```python
from build123d import *


with BuildPart() as part:
    # Sketch1 → Revolve1 (revolve)
    with BuildSketch(Plane.XY):
        with BuildLine():
            Line((-26.9875, 9.525), (26.9875, 9.525))
            Line((26.9875, 9.525), (26.9875, 19.05))
            Line((26.9875, 19.05), (6.112639692, 19.05))
            Line((6.112639692, 19.05), (6.112639692, 56.974587415))
            Line((6.112639692, 56.974587415), (76.2, 88.9))
            Line((76.2, 88.9), (76.2, 139.7))
            ThreePointArc((76.2, 139.7), (61.321024484, 175.621024484), (25.4, 190.5))
            Line((25.4, 190.5), (-25.4, 190.5))
            ThreePointArc((-25.4, 190.5), (-61.321024484, 175.621024484), (-76.2, 139.7))
            Line((-76.2, 139.7), (-76.2, 88.9))
            Line((-76.2, 88.9), (-6.112639692, 56.974587415))
            Line((-6.112639692, 56.974587415), (-6.112639692, 19.05))
            Line((-6.112639692, 19.05), (-26.9875, 19.05))
            Line((-26.9875, 19.05), (-26.9875, 9.525))
        make_face()
    revolve(axis=Axis((-76.2, 0, 0), (1, 0, 0)))


solid = part.part
```
Could you check a few things on this model? Use its own coordinates, in mm. A direction names the side the tool comes from. Coordinates: 2 decimals unless noted, no trailing zeros. Write each loop counter-clockwise with the first axis right and the second up, starting at its lowest first coordinate (ties: lowest second). Pieces come first, ordered by that corner, then holes. Notation, with made-up numbers: (-21, 79) - (-1, 79) arc R20 ccw to (-1, 114) - close; hole circle Ø8 at (64.5, -21). An arc over 180 degrees is marked (long way). Use a Markdown table: item, result.
Q1. Imagine slicing it at D-D (x = 51). List the corners of the cut face in (y, z) for me, and give its area (3 significant figures).
Geometry check:
| item | result |
|---|---|
| outline | circle Ø367.16 at (0, 0); hole circle Ø154.84 at (0, 0) |
| area | 87,000 mm2 |
Q2. Thinking about a two-plate mould opening in Y: for faces 1 (the conical face through (10.5, -12.78, -57.57)), 2 (the flat face through (76.2, 2, -91)), 3 (the conical face through (-9.516, -46.443, -35.611)), 4 (the cylindrical face through (-0.36, -151.17, -115.92)), which applies, +Y half, -Y half, draft (parallel to the pull), parting line (faces both ways), or undercut?
Geometry check:
| item | result |
|---|---|
| face 1 | undercut |
| face 2 | draft |
| face 3 | undercut |
| face 4 | parting line |
Q3. Imagine slicing it at C-C (x = 0.5). List the corners of the cut face in (y, z) for me (3 decimals).
Geometry check:
| item | result |
|---|---|
| outline | circle Ø381 at (0, 0); hole circle Ø19.05 at (0, 0) |
Q4. I'm going to push flat-ended pins straight in: pin 1 Ø19 at (y, z) = (2, 1) entering from -X; pin 2 Ø3 at (x, z) = (29, 138.5) entering from -Y; pin 3 Ø12 at (x, y) = (49.5, 69) entering from +Z. Where does each tip first touch, or does it pass through?
Geometry check:
| item | result |
|---|---|
| pin 1 | stops at x = -26.99 |
| pin 2 | stops at y = -132.19 |
| pin 3 | stops at z = 174.87 |
Q5. Which directions (+Z, -Z, +X, -X, +Y, -Y) give clear straight access to the entire face, cutting with the end or side of a thin tool? Please do faces 5 (the flat face through (-76.2, -2, -91)), 6 (the flat face through (-26.987, 4, 9)), 7 (the flat face through (26.987, -4, 9)).
Geometry check:
| item | result |
|---|---|
| face 5 | +Z, -Z, -X, +Y, -Y |
| face 6 | -X |
| face 7 | +X |
Q6. Please list where these lines run through material, in increasing order: L1, parallel to Z at x = -8.5, y = 0 (3 decimals); L2, parallel to X at y = -7.5, z = -25; L3, parallel to X at y = 9.5, z = 3.5.
Geometry check:
| item | result |
|---|---|
| L1 | z = -190.5 to -58.062, -19.05 to -9.525, 9.525 to 19.05, 58.062 to 190.5 |
| L2 | x = -6.11 to 6.11 |
| L3 | x = -26.99 to 26.99 |
